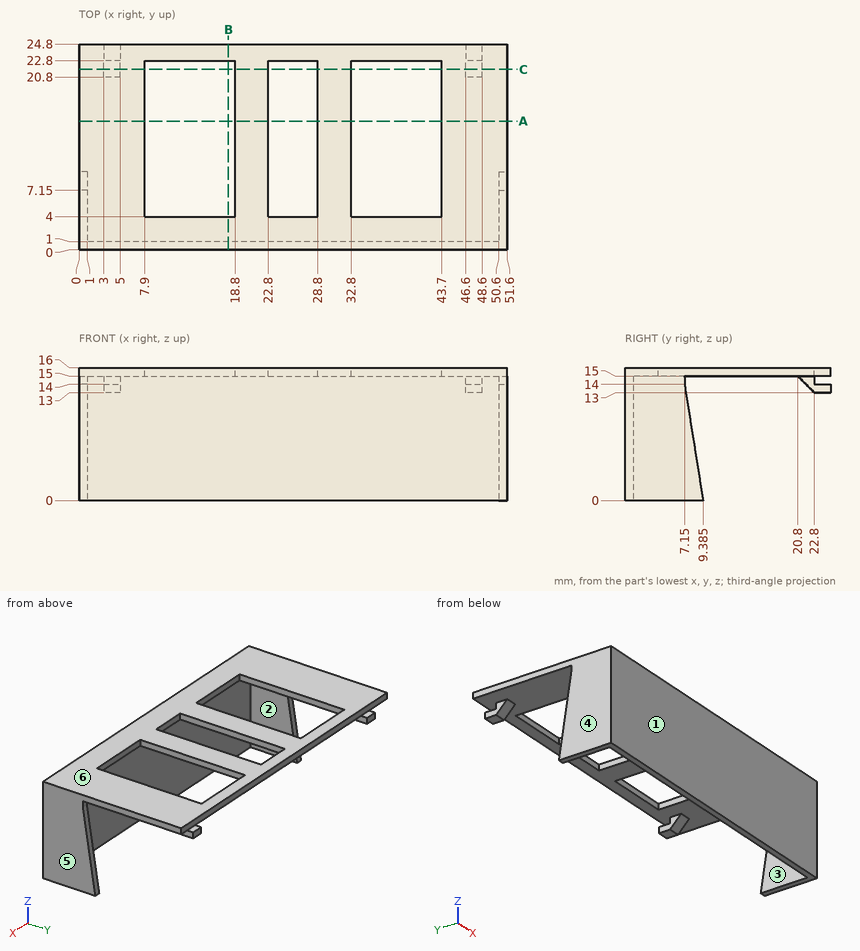
Here's the drawing with two shaded views (mm, measured from the low corner). I have some questions. A direction names the side the tool comes from. Give positions to 0.01 mm unless a question says otherwise; leave off trailing zeros. Order: outer loops, then holes, each group sorted by start corner. A loop starts at its lowest first (then second) coordinate and runs counter-clockwise, first axis right, second up. Notation, with made-up numbers: (78, 78) -> (120, 78) arc R29 cw to (120, 100) -> close; hole circle Ø10 at (50, -38.5). An arc over 180 degrees is marked (long way). Use a Markdown table: item, result. Add a question column.
Item 1: Imagine slicing it at B-B on x = 18. Please give me the cut outline in (y, z), plus the area to 3 significant figures.
Item 2: I need wall thicknesses on line 1 (X direction, y = 6, z = 10.5); line 2 (Y direction, x = 22, z = 7.75); line 3 (Z direction, x = 2, y = 23.25). Which ranges of each line are inside material? Lowest first, please.
Item 3: Imagine slicing it at A-A on y = 15.5. Please give me the cut outline in (x, z), plus the area to 3 significant figures.
Item 4: Will these pins go through, and if not, where does the flat tip stop? pin 1 (0.8 mm diameter, centred on x = 0.5, z = 14.5, fed in from +Y); pin 2 (0.5 mm diameter, centred on x = 47.5, z = 14.5, fed in from +Y); pin 3 (2 mm diameter, centred on y = 23.5, z = 13.5, fed in from +X).
Item 5: Imagine slicing it at C-C on y = 21.75. Please give me the cut outline in (x, z).
Item 6: If we mould it in two halves opening along X, with no side actions, what happens to the marked faces 3, 4, 5 and 6? For each: pulls with the +X half, pulls with the -X half, needs draft (parallel to the pull), parting line crosses it, or undercut.
Item 7: For the marked faces 1 and 2, which set-ups out of +Z, -Z, +X, -X, +Y, -Y let a thin tool reach every point of the face, with its end or its side?
Data:
| question | item | result |
|---|---|---|
| 1 | outline | (0, 0) -> (1, 0) -> (1, 15) -> (4, 15) -> (4, 16) -> (0, 16) -> close; (22.8, 15) -> (24.8, 15) -> (24.8, 16) -> (22.8, 16) -> close |
| 1 | area | 21.0 mm² |
| 2 | line 1 | x = 0 to 1, 50.6 to 51.6 |
| 2 | line 2 | y = 0 to 1 |
| 2 | line 3 | z = 15 to 16 |
| 3 | outline | (0, 15) -> (7.9, 15) -> (7.9, 16) -> (0, 16) -> close; (18.8, 15) -> (22.8, 15) -> (22.8, 16) -> (18.8, 16) -> close; (28.8, 15) -> (32.8, 15) -> (32.8, 16) -> (28.8, 16) -> close; (43.7, 15) -> (51.6, 15) -> (51.6, 16) -> (43.7, 16) -> close |
| 3 | area | 23.8 mm² |
| 4 | pin 1 | stops at y = 7.15 |
| 4 | pin 2 | stops at y = 22.8 |
| 4 | pin 3 | stops at x = 48.6 |
| 5 | outline | (0, 15) -> (3, 15) -> (3, 14.05) -> (5, 14.05) -> (5, 15) -> (7.9, 15) -> (7.9, 16) -> (0, 16) -> close; (18.8, 15) -> (22.8, 15) -> (22.8, 16) -> (18.8, 16) -> close; (28.8, 15) -> (32.8, 15) -> (32.8, 16) -> (28.8, 16) -> close; (43.7, 15) -> (46.6, 15) -> (46.6, 14.05) -> (48.6, 14.05) -> (48.6, 15) -> (51.6, 15) -> (51.6, 16) -> (43.7, 16) -> close |
| 6 | face 3 | undercut |
| 6 | face 4 | pulls with the -X half |
| 6 | face 5 | pulls with the +X half |
| 6 | face 6 | needs draft |
| 7 | face 1 | +Z, -Z, +X, -X, -Y |
| 7 | face 2 | -Z, +Y |
